Check sheet for the modelled part. Datum: model origin and axes. Units: mm. A direction names the side the tool comes from. Give positions to 0.01 mm unless a question says otherwise; leave off trailing zeros. Write each loop counter-clockwise with the first axis right and the second up, starting at its lowest first coordinate (ties: lowest second). Pieces come first, ordered by that corner, then holes. Notation, with made-up numbers: (56.5, 23.5) -> (73.5, 23.5) arc R17 cw to (73.5, 30.5) -> close; hole circle Ø7 at (15, 46.5). An arc over 180 degrees is marked (long way). Write each question's results on one line, items separated by ' | '. Start each with the question number.
```python
from build123d import *

# Parameters (mm, degrees)
SKETCH1_W          = 36.35
SKETCH1_H          = 200
SKETCH1_R          = 1.75
BASE_FLANGE1_DEPTH = 3.175
SKETCH2_W          = 3.175
SKETCH2_H          = 25
CUT_EXTRUDE1_DEPTH = 10
LPATTERN1_COUNT    = 6
LPATTERN1_PITCH    = 40


# Sheet-metal steps are written as plain solids
with BuildPart() as part:
    # Sketch1 → Base-Flange1 (new body)
    with BuildSketch(Plane.XY):
        with Locations((24.256146731, 10.708830738)):
            Rectangle(SKETCH1_W, SKETCH1_H)
        with Locations((24.256146731, 98.208830738)):
            Circle(SKETCH1_R, mode=Mode.SUBTRACT)
        with Locations((24.256146731, 73.208830738)):
            Circle(SKETCH1_R, mode=Mode.SUBTRACT)
        with Locations((24.256146731, 48.208830738)):
            Circle(SKETCH1_R, mode=Mode.SUBTRACT)
        with Locations((24.256146731, 23.208830738)):
            Circle(SKETCH1_R, mode=Mode.SUBTRACT)
        with Locations((24.256146731, -1.791169262)):
            Circle(SKETCH1_R, mode=Mode.SUBTRACT)
        with Locations((24.256146731, -26.791169262)):
            Circle(SKETCH1_R, mode=Mode.SUBTRACT)
        with Locations((24.256146731, -51.791169262)):
            Circle(SKETCH1_R, mode=Mode.SUBTRACT)
        with Locations((24.256146731, -76.791169262)):
            Circle(SKETCH1_R, mode=Mode.SUBTRACT)
    extrude(amount=-BASE_FLANGE1_DEPTH)

    # Sketch2 → Cut-Extrude1 (cut)
    with BuildSketch(Plane.XY):
        with Locations((7.668646731, -89.291169262)):
            Rectangle(SKETCH2_W, SKETCH2_H)
        with Locations((40.843646731, -89.291169262)):
            Rectangle(SKETCH2_W, SKETCH2_H)
    cut_extrude1 = extrude(amount=-CUT_EXTRUDE1_DEPTH, mode=Mode.SUBTRACT)

    # LPattern1: Cut-Extrude1 ×6
    with Locations(*[(0, i * LPATTERN1_PITCH, 0) for i in range(1, LPATTERN1_COUNT)]):
        add(cut_extrude1, mode=Mode.SUBTRACT)


solid = part.part
```
Item 1: Set-up check for faces 4 (the flat face through (8, 83.209, -2)), 5 (the flat face through (41, 43.209, -2)), 6 (the flat face through (41, -76.791, -2)), 7 (the flat face through (6.081, 91, -2)): record each of +Z, -Z, +X, -X, +Y, -Y from which the full face is reachable in a straight line by a thin tool's end or side.
Item 2: Mould release check, pull along Y, two halves, no side actions. Record for faces 1 (the flat face through (41, 98.209, -2)), 2 (the flat face through (39.256, 104, -2)), 3 (the cylindrical face through (25.925, -1.266, -1.565)): pulls with the +Y half, pulls with the -Y half, needs draft (parallel to the pull), parting line crosses it, or undercut.
Item 3: Section check A-A on y = 34. Record the boundary of the cut face in (x, z) (3 decimals).
Item 4: Depth check by flat-ended pin: pin 1 Ø1 at (y, z) = (-80, -2) entering from +X; pin 2 Ø1 at (x, z) = (40.5, -2) entering from -Y; pin 3 Ø4.5 at (x, y) = (24.26, -26.79) entering from +Z; pin 4 Ø1.6 at (x, z) = (40.5, -1) entering from +Y. Enter the tip coordinate at first touch or a pass-through.
Item 5: Section check B-B on z = -1.75. Count the separate pieces of the cut face and the enclosed holes in it, then the cut area to 3 significant figures.
Item 6: Thickness scan on probe 1 along X at (y, z) = (75, -1.65); probe 2 along X at (y, z) = (98.5, -1.85). Record the ranges inside material, lowest first. Write a range as from..to.
Check sheet entries:
1) face 4: +Z, -Z, -X | face 5: +Z, -Z, +X | face 6: +Z, -Z, +X, -Y | face 7: +Z, -Z, -X, +Y, -Y
2) face 1: pulls with the +Y half | face 2: needs draft | face 3: undercut
3) outline: (9.256, -3.175) -> (39.256, -3.175) -> (39.256, 0) -> (9.256, 0) -> close
4) pin 1: stops at x = 39.26 | pin 2: stops at y = -76.79 | pin 3: stops at z = 0 | pin 4: stops at y = 98.21
5) separate pieces: 1 | enclosed holes: 8 | area: 6,400 mm^2
6) probe 1: x = 9.26..39.26 | probe 2: x = 9.26..22.53, 25.98..39.26
